Autodesk Inventor part; units mm, degrees
ref_plane "YZ Plane" through (0, 0, 0) normal (1, 0, 0) x (0, 1, 0)
ref_plane "XZ Plane" through (0, 0, 0) normal (0, 1, 0) x (-1, 0, 0)
ref_plane "XY Plane" through (0, 0, 0) normal (0, 0, 1) x (1, 0, 0)
sketch "스케치1" plane through (0, 0, 0) normal (0, 1, 0) x (-1, 0, 0)
  line L0 (-2.4, 4.8) -> (2.4, 4.8)
  line L1 (2.4, 4.8) -> (2.4, -4.8)
  line L2 (2.4, -4.8) -> (-2.4, -4.8)
  line L3 (-2.4, -4.8) -> (-2.4, 4.8)
  line L4 (-2.4, 4.8) -> (2.4, -4.8) construction
  line L5 (2.4, 4.8) -> (-2.4, -4.8) construction
  point P0 (0, 0)
  dimension "d0" = 4.8
  dimension "d1" = 9.6
extrude "돌출1" add sketch "스케치1" along normal blind 0.6
sketch "스케치2" plane through (0, 0, 0) normal (0, -1, 0) x (1, 0, 0)
  line L0 (2.4, -4.8) -> (-2.4, -4.8)
  line L1 (2.4, 4.8) -> (2.4, -4.8)
  line L2 (-2.4, 4.8) -> (2.4, 4.8)
  line L3 (-2.4, -4.8) -> (-2.4, 4.8)
  line L4 (2.4, 4.8) -> (3, 4.8)
  line L5 (3, 4.8) -> (3, -4.8)
  line L6 (3, -4.8) -> (2.4, -4.8)
  line L7 (2.4, -4.8) -> (2.4, 4.8)
  line L8 (-2.4, -4.8) -> (-2.4, 4.8)
  line L9 (-2.4, 4.8) -> (-3, 4.8)
  line L10 (-3, 4.8) -> (-3, -4.8)
  line L11 (-3, -4.8) -> (-2.4, -4.8)
  line L12 (-2.4, -4.8) -> (-2.4, 4.8)
  point P0 (0, 0)
  dimension "d4" = 0.6
  dimension "d5" = 0.6
extrude "돌출2" add sketch "스케치2" against normal blind 3.1 contours L1 L4 L5 L6 | L11 L10 L9 L3
sketch "스케치3" plane through (0, 0, 0) normal (0, -1, 0) x (1, 0, 0)
  line L0 (2.4, -4.8) -> (-2.4, -4.8)
  line L1 (-0.5, 4.8) -> (0.5, 4.8)
  line L2 (0.5, 4.8) -> (0.5, -4.8)
  line L3 (0.5, -4.8) -> (-0.5, -4.8)
  line L4 (-0.5, -4.8) -> (-0.5, 4.8)
  line L5 (-0.5, 4.8) -> (0.5, -4.8) construction
  line L6 (0.5, 4.8) -> (-0.5, -4.8) construction
  point P0 (0, 0)
  dimension "d8" = 1
extrude "돌출3" add sketch "스케치3" along normal blind 1.8
chamfer "모따기1" distance 1 angle 45 2 edges at (-0.5, 0, 0) (0.5, 0, 0)
sketch "스케치4" plane through (0, -1.8, 0) normal (0, -1, 0) x (1, 0, 0)
  line L0 (1.5, 4.8) -> (0.5, 4.8)
  line L1 (0.5, 4.8) -> (0.5, -4.8)
  line L2 (0.5, -4.8) -> (1.5, -4.8)
  line L3 (1.5, -4.8) -> (1.5, 4.8)
  line L4 (-0.5, 4.8) -> (-0.5, -4.8)
  line L5 (-0.5, -4.8) -> (0.5, -4.8)
  line L6 (0.5, -4.8) -> (0.5, 4.8)
  line L7 (0.5, 4.8) -> (-0.5, 4.8)
  line L8 (-1.5, -4.8) -> (-0.5, -4.8)
  line L9 (-0.5, -4.8) -> (-0.5, 4.8)
  line L10 (-0.5, 4.8) -> (-1.5, 4.8)
  line L11 (-1.5, 4.8) -> (-1.5, -4.8)
  line L12 (-1.5, 1.6) -> (1.5, 1.6)
  line L13 (1.5, 1.6) -> (1.5, -1.6)
  line L14 (1.5, -1.6) -> (-1.5, -1.6)
  line L15 (-1.5, -1.6) -> (-1.5, 1.6)
  line L16 (-1.5, 1.6) -> (1.5, -1.6) construction
  line L17 (1.5, 1.6) -> (-1.5, -1.6) construction
  point P0 (0, 0)
  point P1 (-0.5, -1.6)
  point P2 (-0.5, 1.6)
  point P3 (0.5, -1.6)
  point P4 (0.5, 1.6)
  dimension "d14" = 3.2
extrude "돌출4" cut sketch "스케치4" against normal up to surface (1.8 mm away) contours L3 L14 L1 L12 | L4 L14 L11 L12
properties part number "endcap_4mm_2ea_typeB_ver2_onyx_addon"
Geometry check sheet. Reference: the model listing, model coordinates, mm. A direction names the side the tool comes from. Coordinates: 2 decimals unless noted, no trailing zeros. Loops run counter-clockwise (first coordinate to the right, second up) from the corner with the lowest first, then second, coordinate; pieces in that order, holes last. Notation, with made-up numbers: (60, 48) - (70, 48) arc R22 cw to (70, 86) - close; hole circle Ø6 at (43.5, -39). An arc over 180 degrees is marked (long way). One line per item, written item: value. Start each with the question number.
(1) Tool access check on faces 4 (the flat face through (0, 0.6, 0)), 5 (the flat face through (-2, 0, 0)), 6 (the flat face through (0.5, -1, 0)). Record the directions out of +Z, -Z, +X, -X, +Y, -Y that give a thin tool (end or side, any length) a straight path to the whole face; none if there is none.
(2) Cross-section at D-D on x = 0.85. Enter the section's corners in (y, z), plus the area to 3 significant figures.
(3) Depth check by flat-ended pin: P1, Ø0.9, axis at y = -1, z = -0.5, coming from the -X side; P2, Ø0.8, axis at x = 2, z = -1.5, coming from the -Y side; P3, Ø0.5, axis at y = -1, z = 0, coming from the +X side. Enter the tip coordinate at first touch or a pass-through.
(4) Cross-section at A-A on y = 2.6. Enter the section's corners in (x, z).
(5) Cross-section at B-B on x = -0.7. Enter the section's corners in (y, z), plus the area to 3 significant figures.
(6) Mould release check, pull along X, two halves, no side actions. Record for faces 1 (the flat face through (-1, -0.5, -3.2)), 2 (the flat face through (-2.4, 2, 0)), 3 (the flat face through (0, -1.8, 0)): released by +X, released by -X, zero draft, split by the parting line, or undercut.
(7) Cross-section at C-C on z = 2.5. Enter the section's corners in (x, y), plus the area to 3 significant figures.
(8) Material ranges on line 1 (X direction, y = 2.7, z = 4.25); line 2 (X direction, y = -1.3, z = 2.25); line 3 (Y direction, x = 2.05, z = 1), recorded low to high. Write a range as [from, to].
Results below:
1. face 4: +Z, -Z, +Y
1. face 5: -X, -Y
1. face 6: +X, -Y
2. outline: (-0.65, -4.8) - (0.6, -4.8) - (0.6, 4.8) - (-0.65, 4.8) - (-0.65, 1.6) - (0, 1.6) - (0, -1.6) - (-0.65, -1.6) - close
2. area: 9.92 mm2
3. P1: stops at x = -0.5
3. P2: stops at y = 0
3. P3: stops at x = 0.5
4. outline: (-3, -4.8) - (-2.4, -4.8) - (-2.4, 4.8) - (-3, 4.8) - close; (2.4, -4.8) - (3, -4.8) - (3, 4.8) - (2.4, 4.8) - close
5. outline: (-0.8, -4.8) - (0.6, -4.8) - (0.6, 4.8) - (-0.8, 4.8) - (-0.8, 1.6) - (0, 1.6) - (0, -1.6) - (-0.8, -1.6) - close
5. area: 10.9 mm2
6. face 1: released by -X
6. face 2: undercut
6. face 3: zero draft
7. outline: (-3, 0) - (-1.5, 0) - (-0.5, -1) - (-0.5, -1.8) - (0.5, -1.8) - (0.5, -1) - (1.5, 0) - (3, 0) - (3, 3.1) - (2.4, 3.1) - (2.4, 0.6) - (-2.4, 0.6) - (-2.4, 3.1) - (-3, 3.1) - close
7. area: 9.40 mm2
8. line 1: x = [-3, -2.4], [2.4, 3]
8. line 2: x = [-0.5, 0.5]
8. line 3: y = [0, 0.6]
